from build123d import *

# Parameters (mm, degrees)
SKETCH1_R                  = 24
BOSS_EXTRUDE1_DEPTH        = 14
SKETCH2_R                  = 19.5
CUT_EXTRUDE1_DEPTH         = 10
SKETCH3_R                  = 6
CUT_EXTRUDE2_DEPTH         = 1.5
SKETCH4_R                  = 31
BOSS_EXTRUDE2_DEPTH        = 4
SKETCH5_R                  = 19.5
CUT_EXTRUDE3_DEPTH         = 4
F_3_2_3_2_DIAMETER_HOLE1_D = 3.2


with BuildPart() as part:
    # Sketch1 → Boss-Extrude1 (new body)
    with BuildSketch(Plane(origin=(0, 0, 0), x_dir=(1, 0, 0), z_dir=(0, 1, 0))):
        with Locations(Location((0, 0, 0), (0, 0, 270))):
            Circle(SKETCH1_R)
    extrude(amount=BOSS_EXTRUDE1_DEPTH)

    # Sketch2 → Cut-Extrude1 (cut)
    with BuildSketch(Plane.XZ):
        with Locations(Location((0, 0, 0), (0, 0, 270))):
            Circle(SKETCH2_R)
    extrude(amount=-CUT_EXTRUDE1_DEPTH, mode=Mode.SUBTRACT)

    # Sketch3 → Cut-Extrude2 (cut)
    with BuildSketch(Plane.XZ.offset(-10)):
        with Locations(Location((0, 0, 0), (0, 0, 270))):
            Circle(SKETCH3_R)
    extrude(amount=-CUT_EXTRUDE2_DEPTH, mode=Mode.SUBTRACT)

    # Sketch4 → Boss-Extrude2 (add)
    with BuildSketch(Plane.XZ):
        with Locations(Location((0, 0, 0), (0, 0, 270))):
            Circle(SKETCH4_R)
    extrude(amount=BOSS_EXTRUDE2_DEPTH)

    # Sketch5 → Cut-Extrude3 (cut)
    with BuildSketch(Plane.XZ.offset(4)):
        with Locations(Location((0, 0, 0), (0, 0, 270))):
            Circle(SKETCH5_R)
    extrude(amount=-CUT_EXTRUDE3_DEPTH, mode=Mode.SUBTRACT)

    # Ø3.2 (3.2) Diameter Hole1 (through all)
    with Locations(Plane(origin=(0, 0, 0), x_dir=(1, 0, 0), z_dir=(0, 1, 0))):
        with Locations((-27.5, 0), (0, 27.5), (27.5, 0), (0, -27.5)):
            Hole(F_3_2_3_2_DIAMETER_HOLE1_D / 2)


solid = part.part
For this review, take the finished solid that the model builds, in its own axes (mm). A direction names the side the tool comes from. Round coordinates to 2 decimals unless told otherwise and drop trailing zeros. Write each loop counter-clockwise with the first axis right and the second up, starting at its lowest first coordinate (ties: lowest second). Pieces come first, ordered by that corner, then holes. Notation, with made-up numbers: M 5,-7 L 26,-7 A21 cw 26,1 Z; hole C 21,3 d7. An arc over 180 degrees is marked long. Write item = value, one per line. Start each with the question number.
(1) We need section C-C (x = -27.5). Give the boundary of the cut face in (y, z).
(2) We need section D-D (y = -1). Give the boundary of the cut face in (x, z), then the cut area to 3 significant figures.
(3) Clearance check with flat-ended pins moving along their axes: pin 1 Ø3 at (y, z) = (-1, 7.5) entering from -X; pin 2 Ø4 at (x, y) = (-18.5, 0.5) entering from +Z; pin 3 Ø5 at (y, z) = (4.5, 8.5) entering from -X. State where each tip first meets the part, or that it passes through.
(4) The part is to be moulded in two halves that separate along X. For faces 4 (the face through (7.21, 6.9, 22.89)), 5 (the face through (0.208, -2.028, 25.914)), 6 (the face through (0, -4, -20)), say which applies: +X half, -X half, draft (parallel to the pull), parting line (faces both ways), or undercut.
(5) We need section A-A (x = 0). Give the boundary of the cut face in (y, z), then the cut area to 3 significant figures.
(6) We need section B-B (z = 0). Give the boundary of the cut face in (x, y).
(7) For faces 1 (the face through (7.03, 0, 23.11)), 2 (the face through (0, 14, 0)), 3 (the face through (1.802, 10.74, -5.723)), list the 3-axis set-ups (+Z, -Z, +X, -X, +Y, -Y) from which the entire face can be reached by the end or side of a thin tool; tool diameter is ignored.
(8) For line 1 along Y through (x, z) = (-24.5, 17); line 2 along X through (y, z) = (-1.55, 27.5); line 3 along X through (y, z) = (1.75, 18), list the stretches that pass through material, from the lowest coordinate up.
Results found:
q1.outline = M -4,-14.31 L 0,-14.31 L 0,-1.6 L -4,-1.6 Z; M -4,1.6 L 0,1.6 L 0,14.31 L -4,14.31 Z
q2.outline = C 0,0 d62; hole C -27.5,0 d3.2; hole C 0,0 d39; hole C 0,-27.5 d3.2; hole C 0,27.5 d3.2; hole C 27.5,0 d3.2
q2.area = 1,790 mm²
q3.pin_1 = -30.41
q3.pin_2 = 26.2
q3.pin_3 = -23.24
q4.face_4 = parting line
q4.face_5 = undercut
q4.face_6 = draft
q5.outline = M -4,-31 L 0,-31 L 0,-29.1 L -4,-29.1 Z; M -4,-25.9 L 0,-25.9 L 0,-24 L 14,-24 L 14,24 L 0,24 L 0,25.9 L -4,25.9 L -4,19.5 L 10,19.5 L 10,6 L 11.5,6 L 11.5,-6 L 10,-6 L 10,-19.5 L -4,-19.5 Z; M -4,29.1 L 0,29.1 L 0,31 L -4,31 Z
q5.area = 330 mm²
q6.outline = M -31,-4 L -29.1,-4 L -29.1,0 L -31,0 Z; M -25.9,-4 L -19.5,-4 L -19.5,10 L -6,10 L -6,11.5 L 6,11.5 L 6,10 L 19.5,10 L 19.5,-4 L 25.9,-4 L 25.9,0 L 24,0 L 24,14 L -24,14 L -24,0 L -25.9,0 Z; M 29.1,-4 L 31,-4 L 31,0 L 29.1,0 Z
q7.face_1 = +Y
q7.face_2 = +Z, -Z, +X, -X, +Y
q7.face_3 = -Y
q8.line_1 = -4 to 0
q8.line_2 = -14.31 to -1.6, 1.6 to 14.31
q8.line_3 = -15.87 to -7.5, 7.5 to 15.87
